The figure shows three views and two pictorial views of one solid part (mm, origin at its lowest corner). Answer the questions. A direction names the side the tool comes from. Round coordinates to 2 decimals unless told otherwise and drop trailing zeros. Write each loop counter-clockwise with the first axis right and the second up, starting at its lowest first coordinate (ties: lowest second). Pieces come first, ordered by that corner, then holes.
Item 1: Find section C-C on z = 11.5. Give the vertices of the cut face in (x, y), then the cut area to 3 significant figures.
Item 2: Find the intervals of material crossed by probe 1 along Z at (x, y) = (34, 35); probe 2 along Y at (x, z) = (39, 112); probe 3 along Z at (x, y) = (73.5, 54), in increasing order.
Item 3: A tool of negligible diameter and unlimited length cuts with its end or side. For the marked faces 1 and 2, from which of +Z, -Z, +X, -X, +Y, -Y can it reach the whole face along a straight path? Write none if from no direction.
Item 4: Find section D-D on x = 27.5. Give the vertices of the cut face in (y, z).
Item 5: Find section A-A on y = 40. Give the vertices of the cut face in (x, z).
Item 6: Each of these flat-tipped pins is pushed along its axis until it touches: pin 1 (5 mm diameter, centred on x = 36, z = 28.5, fed in from +Y); pin 2 (12 mm diameter, centred on y = 51, z = 25.5, fed in from +X); pin 3 (6 mm diameter, centred on x = 36, z = 101, fed in from -Y). Where does it stop, or does it pass through?
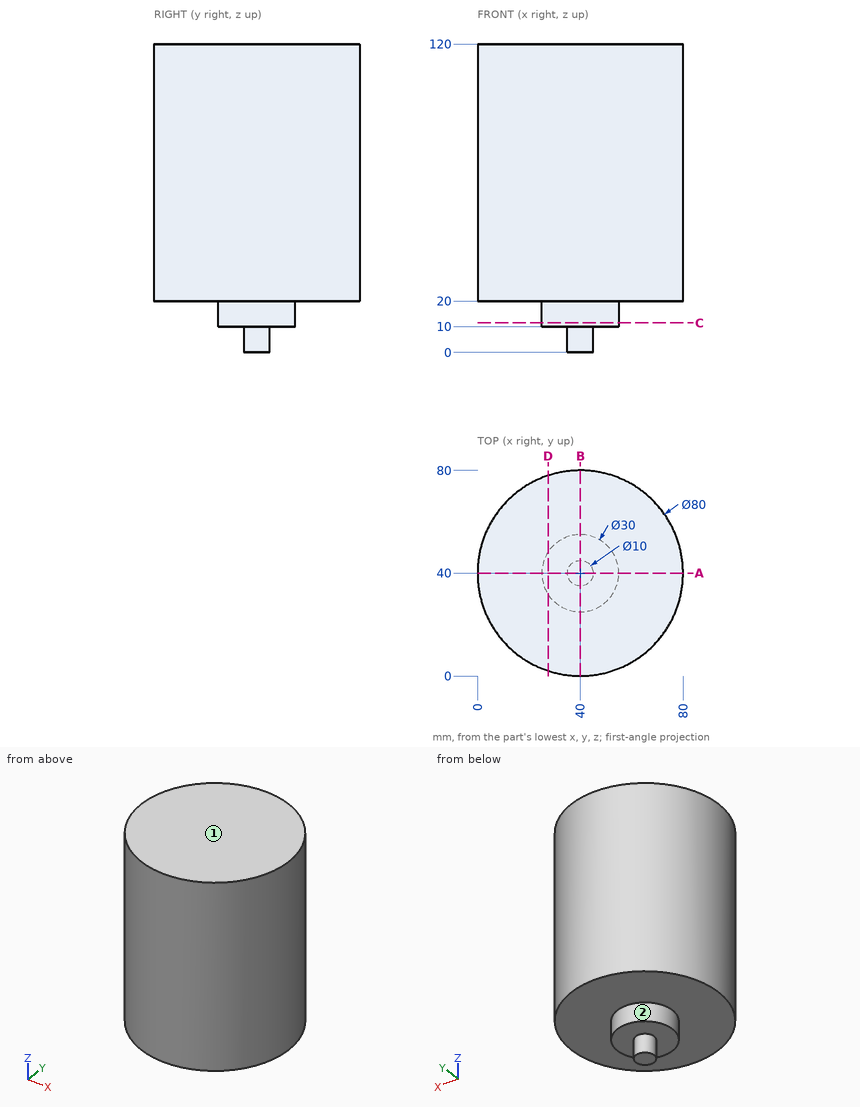
Check values:
1. outline: circle Ø30 at (40, 40)
1. area: 707 mm2
2. probe 1: z = 10 to 120
2. probe 2: y = 0.01 to 79.99
2. probe 3: z = 20 to 120
3. face 1: +Z, +X, -X, +Y, -Y
3. face 2: -Z
4. outline: (2, 20) - (31.71, 20) - (31.71, 10) - (48.29, 10) - (48.29, 20) - (78, 20) - (78, 120) - (2, 120) - close
5. outline: (0, 20) - (25, 20) - (25, 10) - (35, 10) - (35, 0) - (45, 0) - (45, 10) - (55, 10) - (55, 20) - (80, 20) - (80, 120) - (0, 120) - close
6. pin 1: stops at y = 79.97
6. pin 2: stops at x = 79.69
6. pin 3: stops at y = 0.01
